For this review, take the finished solid that the model builds, in its own axes (mm). Face numbers are marked on the shaded views. A direction names the side the tool comes from. Coordinates: 2 decimals unless noted, no trailing zeros. Write each loop counter-clockwise with the first axis right and the second up, starting at its lowest first coordinate (ties: lowest second). Pieces come first, ordered by that corner, then holes. Notation, with made-up numbers: (-39, -38) -> (-2, -38) arc R16 cw to (-2, -11) -> close; hole circle Ø9 at (68, 30.25). An arc over 180 degrees is marked (long way). One line per item, written item: value. Start each with the question number.
1) Add section B-B (z = -37). State the section outline as (x, y) points.
2) Machinability: for the marked faces 1, 2, 3, 4 and 5, which of the approach directions +Z, -Z, +X, -X, +Y, -Y give a long, thin tool a straight path to every point of the face, cutting with its end or side? Answer none if there is none.
3) Add section A-A (y = 10). State the section outline as (x, z) points.
4) Add section C-C (z = -5). State the section outline as (x, y) points, and give its area (3 significant figures).
5) Add section D-D (x = -15). State the section outline as (y, z) points, and give its area (3 significant figures).
6) For pin 1 Ø12 at (x, z) = (-25.5, -36) entering from -Y; pin 2 Ø10 at (x, y) = (-27.5, 48.5) entering from +Z; pin 3 Ø3 at (x, z) = (-3, -7.5) entering from +Y, all flat-tipped, find the tip position at first contact; note any pin that passes through.
7) For probe 1 along Y at (x, z) = (-2.05, -37); probe 2 along Z at (x, y) = (-2.5, 55.5); probe 3 along X at (y, z) = (34.5, -10), list the stretches that pass through material, from the lowest coordinate up. Write a range as from..to.
from build123d import *

# Parameters (mm, degrees)
SKETCH1_W           = 42
SKETCH1_H           = 40
SKETCH1_R           = 2.75
BOSS_EXTRUDE1_DEPTH = 4
BOSS_EXTRUDE2_DEPTH = 20


with BuildPart() as part:
    # Sketch1 → Boss-Extrude1 (new body)
    with BuildSketch(Plane(origin=(0, 0, 0), x_dir=(0, 0, -1), z_dir=(1, 0, 0))):
        with Locations((21, 20)):
            Rectangle(SKETCH1_W, SKETCH1_H)
        with Locations((5, 30)):
            Circle(SKETCH1_R, mode=Mode.SUBTRACT)
        with Locations((5, 10)):
            Circle(SKETCH1_R, mode=Mode.SUBTRACT)
        with Locations((37, 10)):
            Circle(SKETCH1_R, mode=Mode.SUBTRACT)
        with Locations((37, 30)):
            Circle(SKETCH1_R, mode=Mode.SUBTRACT)
    extrude(amount=-BOSS_EXTRUDE1_DEPTH)

    # Sketch3 → Boss-Extrude2 (add)
    with BuildSketch(Plane(origin=(0, 40, 0), x_dir=(1, 0, 0), z_dir=(0, 1, 0))):
        Polygon((0, 42), (-44, 42), (-44, 31.25), (-4, 31.25), (-4, 11), (0, 11), align=None)
    extrude(amount=BOSS_EXTRUDE2_DEPTH)


solid = part.part
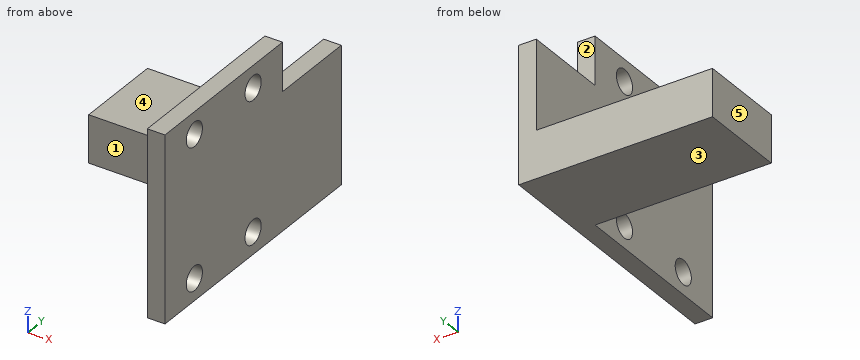
Numbers:
1. outline: (-44, 40) -> (-4, 40) -> (-4, 32.75) -> (0, 32.75) -> (0, 60) -> (-44, 60) -> close; (-4, 0) -> (0, 0) -> (0, 7.25) -> (-4, 7.25) -> close; (-4, 12.75) -> (0, 12.75) -> (0, 27.25) -> (-4, 27.25) -> close
2. face 1: +Z, -Z, -X, -Y
2. face 2: +Z, +X, -X, +Y
2. face 3: -Z, +X, -X, +Y, -Y
2. face 4: +Z, -X, +Y, -Y
2. face 5: +Z, -Z, -X, +Y, -Y
3. outline: (-4, -42) -> (0, -42) -> (0, -39.75) -> (-4, -39.75) -> close; (-4, -34.25) -> (0, -34.25) -> (0, -7.75) -> (-4, -7.75) -> close; (-4, -2.25) -> (0, -2.25) -> (0, 0) -> (-4, 0) -> close
4. outline: (-4, 0) -> (0, 0) -> (0, 7.25) -> (-4, 7.25) -> close; (-4, 12.75) -> (0, 12.75) -> (0, 27.25) -> (-4, 27.25) -> close; (-4, 32.75) -> (0, 32.75) -> (0, 40) -> (-4, 40) -> close
4. area: 116 mm²
5. outline: (40, -42) -> (60, -42) -> (60, -31.25) -> (40, -31.25) -> close
5. area: 215 mm²
6. pin 1: y = 40
6. pin 2: z = -31.25
6. pin 3: y = 40
7. probe 1: 0..7.25, 12.75..27.25, 32.75..60
7. probe 2: -42..-11
7. probe 3: -4..0
